The figure shows three views and two pictorial views of one solid part (mm, origin at its lowest corner). Answer the questions. Coordinates: 2 decimals unless noted, no trailing zeros. Order: outer loops, then holes, each group sorted by start corner. A loop starts at its lowest first (then second) coordinate and runs counter-clockwise, first axis right, second up. Notation, with made-up numbers: (-38.5, 18) -> (-24.5, 18) arc R30 cw to (-24.5, 41) -> close; hole circle Ø11 at (88.25, 20.5). An arc over 180 degrees is marked (long way). Write item = value, one per line. Start each with the question number.
Q1. Straight lines are drawn through the part: L1, parallel to X at y = 1.9, z = 3.75; L2, parallel to Z at x = 9.5, y = 3.1; L3, parallel to Z at x = 3.5, y = 3.15. For each, find the intervals that lie inside material, in ascending order. Write a range as from..to.
Q2. The part is cut by section C-C, the plane x = 6.75. Determine the outline of the cut face in (y, z).
Q3. The part is cut by section B-B, the plane y = 2.7. Determine the outline of the cut face in (x, z).
Q4. The part is cut by section A-A, the plane z = 6.5. Determine the outline of the cut face in (x, y), plus the area to 3 significant figures.
Q5. Flat-ended cylindrical pins translate along their axes: pin 1 (1.5 mm diameter, centred on x = 6, y = 1.5, fed in from +Z); pin 2 (3 mm diameter, centred on y = 1, z = 7, fed in from +X); pin 3 (2 mm diameter, centred on y = 4, z = 8.5, fed in from +X). Find the tip coordinate at first contact, or state that the pin passes through.
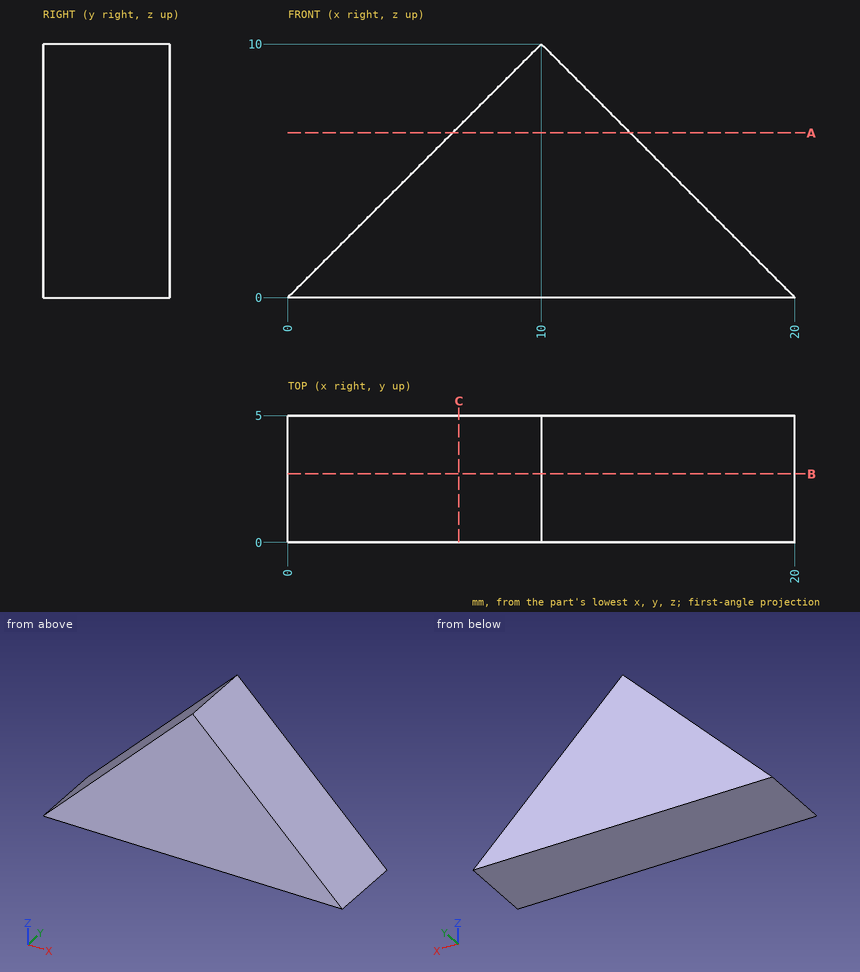
Model answer:
q1.L1 = 3.75..16.25
q1.L2 = 0..9.5
q1.L3 = 0..3.5
q2.outline = (0, 0) -> (5, 0) -> (5, 6.75) -> (0, 6.75) -> close
q3.outline = (0, 0) -> (20, 0) -> (10, 10) -> close
q4.outline = (6.5, 0) -> (13.5, 0) -> (13.5, 5) -> (6.5, 5) -> close
q4.area = 35.0 mm2
q5.pin_1 = 6.75
q5.pin_2 = 14.5
q5.pin_3 = 12.5
